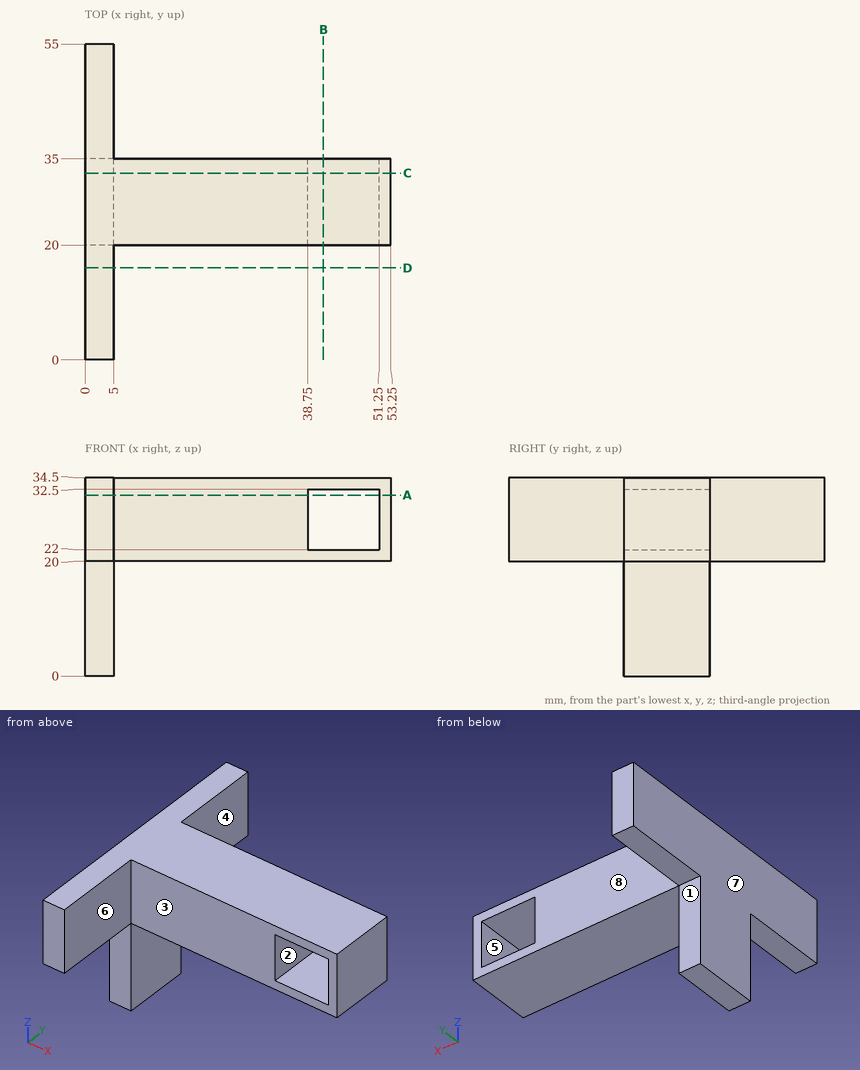
Study the drawing (mm; zero at the part's minimum x, y, z) and answer. A direction names the side the tool comes from. Coordinates: 2 decimals unless noted, no trailing zeros. Loops run counter-clockwise (first coordinate to the right, second up) from the corner with the lowest first, then second, coordinate; pieces in that order, holes last. Notation, with made-up numbers: (-17.5, 1.25) -> (-0.5, 1.25) arc R32 cw to (-0.5, 34.25) -> close; hole circle Ø3 at (-5, -21). An arc over 180 degrees is marked (long way). Write item = value, one per line. Start each with the question number.
1) The part is cut by section A-A, the plane z = 31.5. Determine the outline of the cut face in (x, y), plus the area to 3 significant figures.
2) The part is cut by section D-D, the plane y = 16. Determine the outline of the cut face in (x, z).
3) For the marked faces 1, 2, 3 and 4, determine the directions among +Z, -Z, +X, -X, +Y, -Y from which every point of the face is accessible in a straight line to the end or side of a thin tool.
4) The mould has two halves that part along X. Classify the marked faces 5, 6, 7 and 8: pulls with the +X half, pulls with the -X half, needs draft (parallel to the pull), parting line crosses it, or undercut.
5) The part is cut by section B-B, the plane x = 41.5. Determine the outline of the cut face in (y, z), plus the area to 3 significant figures.
6) Find the intervals of material crossed by L1, parallel to X at y = 32.5, z = 29.5; L2, parallel to X at y = 37, z = 31; L3, parallel to Y at x = 34, z = 27, in increasing order. Write a range as from..to.
7) The part is cut by section C-C, the plane y = 32.5. Determine the outline of the cut face in (x, z).
8) Given P1, Ø6, axis at x = 42.5, y = 26, coming from the -Z side; P2, Ø2.5, axis at x = 1.5, z = 9, coming from the -Y side; P3, Ø7, axis at y = 9.5, z = 29.5, coming from the +X side, each flat-ended and moving along its own axis, determine where each tip first touches the part or whether it passes through.
Result:
q1.outline = (0, 0) -> (5, 0) -> (5, 20) -> (38.75, 20) -> (38.75, 35) -> (5, 35) -> (5, 55) -> (0, 55) -> close; (51.25, 20) -> (53.25, 20) -> (53.25, 35) -> (51.25, 35) -> close
q1.area = 811 mm²
q2.outline = (0, 20) -> (5, 20) -> (5, 34.5) -> (0, 34.5) -> close
q3.face_1 = -Z, +X, -X, +Y
q3.face_2 = +Y, -Y
q3.face_3 = +Z, -Z, +X, -Y
q3.face_4 = +Z, -Z, +X, +Y
q4.face_5 = undercut
q4.face_6 = pulls with the +X half
q4.face_7 = pulls with the -X half
q4.face_8 = needs draft
q5.outline = (20, 20) -> (35, 20) -> (35, 22) -> (20, 22) -> close; (20, 32.5) -> (35, 32.5) -> (35, 34.5) -> (20, 34.5) -> close
q5.area = 60.0 mm²
q6.L1 = 0..38.75, 51.25..53.25
q6.L2 = 0..5
q6.L3 = 20..35
q7.outline = (0, 0) -> (5, 0) -> (5, 20) -> (53.25, 20) -> (53.25, 34.5) -> (0, 34.5) -> close; hole (38.75, 22) -> (51.25, 22) -> (51.25, 32.5) -> (38.75, 32.5) -> close
q8.P1 = 20
q8.P2 = 20
q8.P3 = 5
